Input: part model. Units: mm. Frame: model coordinates. Face numbers are marked on the shaded views. A direction names the side the tool comes from. Round coordinates to 2 decimals unless told otherwise and drop trailing zeros. Loops run counter-clockwise (first coordinate to the right, second up) from the corner with the lowest first, then second, coordinate; pieces in that order, holes last.
(1) First-contact query: pin 1 Ø5 at (y, z) = (-12.5, 13) entering from +X; pin 2 Ø10 at (y, z) = (-2, 16.5) entering from +X; pin 3 Ø1.5 at (y, z) = (-10.5, 16) entering from -X; pin 4 Ø12 at (y, z) = (12, 2) entering from -X. Flat tips, straight axial feed; report the tip coordinate or a pass-through.
(2) Access query for the marked faces 4, 5 and 6. Directions: +Z, -Z, +X, -X, +Y, -Y. A direction counts if a zero-diameter tool reaches every point of the face in a straight line with its end or side. Return the directions, or none.
(3) Cut plane B-B, the plane z = 13. Output: boundary loops of the cut face in (x, y), and give its area (3 significant figures).
(4) Cut plane C-C, the plane y = 6. Output: boundary loops of the cut face in (x, z).
(5) Draft query along Y for the marked faces 1, 2 and 3. Return one class per face: released by +Y, released by -Y, zero draft, split by the parting line, or undercut.
(6) Line query: line 1 (Z direction, x = 1, y = -15); line 2 (Z direction, x = 10.75, y = 6.5); line 3 (Y direction, x = -0.75, z = 18). Output: solid intervals per line, ascending.
(7) Cut plane D-D, the plane x = 8. Output: boundary loops of the cut face in (y, z), and give its area (3 significant figures).
(8) Cut plane A-A, the plane x = -4. Output: boundary loops of the cut face in (y, z), and give its area (3 significant figures).
Autodesk Inventor part; units mm, degrees
ref_plane "YZ Plane" through (0, 0, 0) normal (1, 0, 0) x (0, 1, 0)
ref_plane "XZ Plane" through (0, 0, 0) normal (0, 1, 0) x (-1, 0, 0)
ref_plane "XY Plane" through (0, 0, 0) normal (0, 0, 1) x (1, 0, 0)
sketch "Sketch1" plane through (0, 0, 0) normal (0, 0, 1) x (1, 0, 0)
  circle A0 centre (0, 0) radius 12.7
  line L0 (-10.95, 6.4333) -> (-10.95, -6.4333)
  dimension "d0" = 25.4
  dimension "d1" = 23.65
extrude "Extrusion1" add sketch "Sketch1" along normal blind 19 contours A0 L0 picked at (-3.0667, 0)
sketch "Sketch2" plane through (0, 0, 0) normal (0, 0, -1) x (-1, 0, 0)
  line L0 (0, 16.5122) -> (14.3, 8.2561)
  line L1 (14.3, 8.2561) -> (14.3, -8.2561)
  line L2 (14.3, -8.2561) -> (0, -16.5122)
  line L3 (0, -16.5122) -> (-14.3, -8.2561)
  line L4 (-14.3, -8.2561) -> (-14.3, 8.2561)
  line L5 (-14.3, 8.2561) -> (0, 16.5122)
  point P0 (0, 0)
  point P1 (0, 0)
  dimension "d5" = 28.6
extrude "Extrusion2" add sketch "Sketch2" along normal blind 2.5
sketch "Sketch3" plane through (0, 0, 19) normal (0, 0, 1) x (1, 0, 0)
  circle A0 centre (0, 0) radius 10.95
  arc A1 (-10.95, -6.4333) -> (-10.95, 6.4333) centre (0, 0) ccw
  line L0 (-10.95, 6.4333) -> (-10.95, -6.4333)
  point P0 (-10.95, 0)
extrude "Extrusion3" cut sketch "Sketch3" against normal blind 5
sketch "Sketch4" plane through (0, 0, 19) normal (0, 0, 1) x (1, 0, 0)
  line L0 (-7, 3) -> (7, 3)
  line L1 (7, 3) -> (7, -3)
  line L2 (7, -3) -> (-7, -3)
  line L3 (-7, -3) -> (-7, 3)
  point P0 (0, 0)
  point P1 (7, 0)
  point P2 (0, 3)
  dimension "d10" = 14
  dimension "d11" = 6
extrude "Extrusion4" cut sketch "Sketch4" against normal blind 5
thread "Thread1"
properties part number "RS PRO USB 2.0 Cable, Female USB A to Male USB A USB Extension Cable, 200mm"
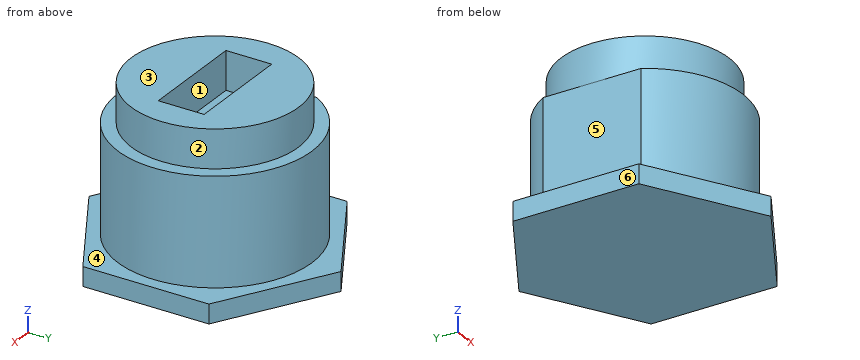
Reported:
1. pin 1: stops at x = 7.83
1. pin 2: stops at x = 12.7
1. pin 3: stops at x = -4.98
1. pin 4: stops at x = -14.3
2. face 4: +Z
2. face 5: +Z, -X, +Y, -Y
2. face 6: +Z, -Z, -X, +Y, -Y
3. outline: (-10.95, -6.43) arc R12.7 ccw (long way) to (-10.95, 6.43) - close
3. area: 491 mm2
4. outline: (-14.3, -2.5) - (14.3, -2.5) - (14.3, 0) - (11.19, 0) - (11.19, 14) - (9.16, 14) - (9.16, 19) - (-9.16, 19) - (-9.16, 14) - (-10.95, 14) - (-10.95, 0) - (-14.3, 0) - close
5. face 1: undercut
5. face 2: split by the parting line
5. face 3: zero draft
6. line 1: z = -2.5 to 0
6. line 2: z = -2.5 to 14
6. line 3: y = -10.92 to -3, 3 to 10.92
7. outline: (-11.89, -2.5) - (11.89, -2.5) - (11.89, 0) - (9.86, 0) - (9.86, 14) - (7.48, 14) - (7.48, 19) - (-7.48, 19) - (-7.48, 14) - (-9.86, 14) - (-9.86, 0) - (-11.89, 0) - close
7. area: 410 mm2
8. outline: (-14.2, -2.5) - (14.2, -2.5) - (14.2, 0) - (12.05, 0) - (12.05, 14) - (10.19, 14) - (10.19, 19) - (3, 19) - (3, 14) - (-3, 14) - (-3, 19) - (-10.19, 19) - (-10.19, 14) - (-12.05, 14) - (-12.05, 0) - (-14.2, 0) - close
8. area: 480 mm2
